The listing builds one solid part. Answer for the finished solid, in the listing's coordinates (mm). Face numbers are marked on the shaded views. A direction names the side the tool comes from. Give positions to 0.01 mm unless a question says otherwise; leave off trailing zeros. Write each loop counter-clockwise with the first axis right and the second up, starting at its lowest first coordinate (ties: lowest second). Pieces come first, ordered by that corner, then holes. Notation, with made-up numbers: M 83.25,31.5 L 105.25,31.5 A7 cw 105.25,38.5 Z; hole C 75,-27.5 d3. An arc over 180 degrees is marked long. Return JSON: item names as keys, results as strings.
from build123d import *

# Parameters (mm, degrees)
SKETCH1_W                                            = 59.1
SKETCH1_H                                            = 59.1
BOSS_EXTRUDE1_DEPTH                                  = 59.1
CUT_EXTRUDE1_START                                   = -2.25
SKETCH2_W                                            = 116.357411776
SKETCH2_H                                            = 94.431830133
CUT_EXTRUDE1_DEPTH                                   = 71.232302632
FILLET1_R                                            = 7.5
SHELL1_T                                             = -2.5
CUT_EXTRUDE7_DEPTH                                   = 35
BOSS_EXTRUDE2_START                                  = 3
SKETCH18_R                                           = 5
BOSS_EXTRUDE2_DEPTH                                  = 3
SKETCH17_R                                           = 1.5
CUT_EXTRUDE10_DEPTH                                  = 10
CUT_EXTRUDE11_REACH                                  = 90.65
CSK_SLOT_FOR_M2_COUNTERSUNK_FLAT_HEAD_SC_D           = 2.4
CSK_SLOT_FOR_M2_COUNTERSUNK_FLAT_HEAD_SC_CSINK_D     = 4.4
CSK_SLOT_FOR_M2_COUNTERSUNK_FLAT_HEAD_SC_CSINK_ANGLE = 90
CSK_SLOT_FOR_M2_COUNTERSUNK_FLAT_HEA_2_D             = 2.4
CSK_SLOT_FOR_M2_COUNTERSUNK_FLAT_HEA_2_CSINK_D       = 4.4
CSK_SLOT_FOR_M2_COUNTERSUNK_FLAT_HEA_2_CSINK_ANGLE   = 90
CSK_SLOT_FOR_M2_COUNTERSUNK_FLAT_HEA_3_D             = 2.4
CSK_SLOT_FOR_M2_COUNTERSUNK_FLAT_HEA_3_CSINK_D       = 4.4
CSK_SLOT_FOR_M2_COUNTERSUNK_FLAT_HEA_3_CSINK_ANGLE   = 90
BOSS_EXTRUDE3_DEPTH                                  = 35
SKETCH28_W                                           = 7.5
SKETCH28_H                                           = 5.1
CUT_EXTRUDE12_DEPTH                                  = 62.984090748
SKETCH29_W                                           = 27.5
SKETCH29_H                                           = 5
BOSS_EXTRUDE4_DEPTH                                  = 5


with BuildPart() as part:
    # Sketch1 → Boss-Extrude1 (new body)
    with BuildSketch(Plane.XY):
        Rectangle(SKETCH1_W, SKETCH1_H)
    extrude(amount=BOSS_EXTRUDE1_DEPTH)

    # Sketch2 → Cut-Extrude1 (cut, through all)
    with BuildSketch(Plane(origin=(-13.400446417, -13.400446417, 19.55), x_dir=(0.9659258262890684, -0.2588190451025203, 0), z_dir=(0, 0, 1)).offset(CUT_EXTRUDE1_START)):
        with Locations((15.241895832, 15.980077556)):
            Rectangle(SKETCH2_W, SKETCH2_H)
    extrude(amount=-CUT_EXTRUDE1_DEPTH, mode=Mode.SUBTRACT)

    # Fillet1
    fillet1_edges = [part.edges().sort_by_distance(p)[0] for p in [
        (29.55, 0, 59.1),
        (0, 29.55, 59.1),
        (-29.55, 0, 59.1),
        (0, -29.55, 59.1),
        (-29.55, 29.55, 38.2),
        (29.55, 29.55, 38.2),
        (29.55, -29.55, 38.2),
        (-29.55, -29.55, 38.2),
    ]]
    fillet(fillet1_edges, radius=FILLET1_R)

    # Shell1
    shell1_openings = [part.faces().sort_by_distance(p)[0] for p in [
        (0, 0, 17.3),
    ]]
    offset(amount=SHELL1_T, openings=shell1_openings, kind=Kind.INTERSECTION)

    # Sketch14 → Cut-Extrude7 (cut)
    with BuildSketch(Plane.XY.offset(59.1)):
        Polygon((-29.55, -8.7), (-27.05, -8.7), (-27.05, -7.5), (-24.55, -7.5), (-24.55, -12.5), (-27.05, -12.5), (-27.05, -11.3), (-29.55, -11.3), align=None)
        Polygon((-29.55, 11.3), (-29.55, 8.7), (-27.05, 8.7), (-27.05, 7.5), (-24.55, 7.5), (-24.55, 12.5), (-27.05, 12.5), (-27.05, 11.3), align=None)
    extrude(amount=-CUT_EXTRUDE7_DEPTH, mode=Mode.SUBTRACT)

    # Sketch18 → Boss-Extrude2 (add)
    with BuildSketch(Plane(origin=(0, -27.05, 0), x_dir=(1, 0, 0), z_dir=(0, 1, 0)).offset(BOSS_EXTRUDE2_START)):
        with Locations((-22.05, -51.6)):
            Circle(SKETCH18_R)
    extrude(amount=-BOSS_EXTRUDE2_DEPTH)

    # Sketch17 → Cut-Extrude10 (cut)
    with BuildSketch(Plane.XZ.offset(29.55)):
        with Locations(Location((-22.05, 51.6, 0), (0, 0, 90))):
            Circle(SKETCH17_R)
    extrude(amount=-CUT_EXTRUDE10_DEPTH, mode=Mode.SUBTRACT)

    # Sketch20 → Cut-Extrude11 (cut, up to next)
    with BuildSketch(Plane.XZ.offset(29.55), mode=Mode.PRIVATE) as cut_extrude11_sk1:
        with BuildLine():
            Line((-22.647878988, 52.975696447), (-23.072143057, 53.399960516))
            Line((-23.072143057, 53.399960516), (-23.849960516, 52.622143057))
            Line((-23.849960516, 52.622143057), (-23.425696447, 52.197878988))
            ThreePointArc((-23.425696447, 52.197878988), (-23.110660172, 52.660660172), (-22.647878988, 52.975696447))
        make_face()
    cut_extrude11_tool1 = extrude(cut_extrude11_sk1.sketch, amount=-CUT_EXTRUDE11_REACH, mode=Mode.PRIVATE) & part.part
    # Sketch20 → Cut-Extrude11 (cut, up to next)
    with BuildSketch(Plane.XZ.offset(29.55), mode=Mode.PRIVATE) as cut_extrude11_sk2:
        with BuildLine():
            Line((-21.027856943, 49.800039484), (-21.452121012, 50.224303553))
            ThreePointArc((-21.452121012, 50.224303553), (-20.989339828, 50.539339828), (-20.674303553, 51.002121012))
            Line((-20.674303553, 51.002121012), (-20.250039484, 50.577856943))
            Line((-20.250039484, 50.577856943), (-21.027856943, 49.800039484))
        make_face()
    cut_extrude11_tool2 = extrude(cut_extrude11_sk2.sketch, amount=-CUT_EXTRUDE11_REACH, mode=Mode.PRIVATE) & part.part
    add(cut_extrude11_tool1.solids().sort_by_distance((-23.27308, -29.55, 52.82308))[0], mode=Mode.SUBTRACT)
    add(cut_extrude11_tool2.solids().sort_by_distance((-20.82692, -29.55, 50.37692))[0], mode=Mode.SUBTRACT)

    # CSK SLOT for M2 Countersunk Flat Head Sc (through all)
    with Locations(Plane.ZX.offset(29.55)):
        with Locations((29.55, 0)):
            CounterSinkHole(CSK_SLOT_FOR_M2_COUNTERSUNK_FLAT_HEAD_SC_D / 2, CSK_SLOT_FOR_M2_COUNTERSUNK_FLAT_HEAD_SC_CSINK_D / 2, counter_sink_angle=CSK_SLOT_FOR_M2_COUNTERSUNK_FLAT_HEAD_SC_CSINK_ANGLE)

    # CSK SLOT for M2 Countersunk Flat Hea 2 (through all)
    with Locations(Plane.XY.offset(59.1)):
        with Locations((0, 0)):
            CounterSinkHole(CSK_SLOT_FOR_M2_COUNTERSUNK_FLAT_HEA_2_D / 2, CSK_SLOT_FOR_M2_COUNTERSUNK_FLAT_HEA_2_CSINK_D / 2, counter_sink_angle=CSK_SLOT_FOR_M2_COUNTERSUNK_FLAT_HEA_2_CSINK_ANGLE)

    # CSK SLOT for M2 Countersunk Flat Hea 3 (through all)
    with Locations(Plane(origin=(0, -29.55, 0), x_dir=(-1, 0, 0), z_dir=(0, -1, 0))):
        with Locations((0, -29.55)):
            CounterSinkHole(CSK_SLOT_FOR_M2_COUNTERSUNK_FLAT_HEA_3_D / 2, CSK_SLOT_FOR_M2_COUNTERSUNK_FLAT_HEA_3_CSINK_D / 2, counter_sink_angle=CSK_SLOT_FOR_M2_COUNTERSUNK_FLAT_HEA_3_CSINK_ANGLE)

    # Sketch27 → Boss-Extrude3 (add)
    with BuildSketch(Plane(origin=(-29.55, 29.55, 0), x_dir=(0, 0, -1), z_dir=(1, 0, 0))):
        Polygon((-18.3, -59.1), (-18.3, -61.7), (-17.05, -61.7), (-17.05, -64.2), (-22.05, -64.2), (-22.05, -61.7), (-20.8, -61.7), (-20.8, -59.1), align=None)
        Polygon((-38.3, -59.1), (-40.8, -59.1), (-40.8, -61.7), (-42.05, -61.7), (-42.05, -64.2), (-37.05, -64.2), (-37.05, -61.7), (-38.3, -61.7), align=None)
    extrude(amount=BOSS_EXTRUDE3_DEPTH)

    # Sketch28 → Cut-Extrude12 (cut, through all)
    with BuildSketch(Plane.XY.offset(59.1)):
        with Locations((-25.8, -32.1)):
            Rectangle(SKETCH28_W, SKETCH28_H)
    extrude(amount=-CUT_EXTRUDE12_DEPTH, mode=Mode.SUBTRACT)

    # Sketch29 → Boss-Extrude4 (add)
    with BuildSketch(Plane.XY.offset(59.1)):
        with Locations((8.3, -10)):
            Rectangle(SKETCH29_W, SKETCH29_H)
        with Locations((8.3, 10)):
            Rectangle(SKETCH29_W, SKETCH29_H)
    extrude(amount=BOSS_EXTRUDE4_DEPTH)


solid = part.part
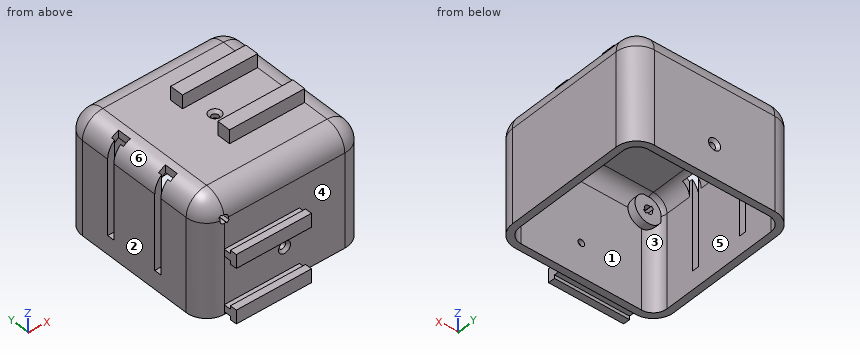
Item 1: Which of the six approach directions +Z, -Z, +X, -X, +Y, -Y give full straight-line access (tool end or side, diameter ignored) to the marked faces 1 and 2?
Geometry results:
{"face 1": "-Z", "face 2": "+Z, -Z, -X, +Y, -Y"}
Item 2: Given pin 1 Ø3 at (x, z) = (0, 29.55) entering from -Y; pin 2 Ø2 at (x, y) = (19.5, -26.5) entering from -Z; pin 3 Ø4 at (x, z) = (-4.5, 51) entering from -Y, each flat-ended and moving along its own axis, determine where each tip first touches the part or whether it passes through.
Geometry results:
{"pin 1": "stops at y = -28.85", "pin 2": "stops at z = 17.3", "pin 3": "stops at y = -29.55"}
Item 3: Determine the mould class of the marked faces 3, 4, 5 and 6 for opening direction X: +X half, -X half, draft (parallel to the pull), parting line (faces both ways), or undercut.
Geometry results:
{"face 3": "undercut", "face 4": "draft", "face 5": "undercut", "face 6": "-X half"}
Item 4: A cutting plane is placed at C-C, the plane x = -15.5. Write down the section's boundary in (y, z).
Geometry results:
{"outline": "M -34.65,17.05 L -32.15,17.05 L -32.15,18.3 L -29.55,18.3 L -29.55,17.3 L -27.05,17.3 L -27.05,51.6 A5 cw -22.05,56.6 L 22.05,56.6 A5 cw 27.05,51.6 L 27.05,17.3 L 29.55,17.3 L 29.55,51.6 A7.5 ccw 22.05,59.1 L -22.05,59.1 A7.5 ccw -29.55,51.6 L -29.55,40.8 L -32.15,40.8 L -32.15,42.05 L -34.65,42.05 L -34.65,37.05 L -32.15,37.05 L -32.15,38.3 L -29.55,38.3 L -29.55,20.8 L -32.15,20.8 L -32.15,22.05 L -34.65,22.05 Z"}
Item 5: A cutting plane is placed at A-A, the plane z = 44. Write down the section's boundary in (x, y), plus the area to 3 significant figures.
Geometry results:
{"outline": "M -29.55,-22.05 A7.5 ccw -22.05,-29.55 L 22.05,-29.55 A7.5 ccw 29.55,-22.05 L 29.55,22.05 A7.5 ccw 22.05,29.55 L -22.05,29.55 A7.5 ccw -29.55,22.05 L -29.55,11.3 L -27.05,11.3 L -27.05,22.05 A5 cw -22.05,27.05 L 22.05,27.05 A5 cw 27.05,22.05 L 27.05,-22.05 A5 cw 22.05,-27.05 L -22.05,-27.05 A5 cw -27.05,-22.05 L -27.05,-11.3 L -29.55,-11.3 Z; M -29.55,-8.7 L -27.05,-8.7 L -27.05,8.7 L -29.55,8.7 Z", "area": "526 mm2"}
Item 6: Find the intervals of material crossed by line 1 (Y direction, x = -21, z = 38); line 2 (X direction, y = 8, z = 38), in increasing order.
Geometry results:
{"line 1": "y = -34.65 to -32.15, -29.55 to -27.05, 27.05 to 29.55", "line 2": "x = -29.55 to -27.05, 27.05 to 29.55"}
Item 7: A cutting plane is placed at D-D, the plane x = 0. Count the separate pieces of the cut face and the enclosed holes in it, plus the area to 3 significant figures.
Geometry results:
{"separate pieces": "4", "enclosed holes": "0", "area": "398 mm2"}
Item 8: A cutting plane is placed at B-B, the plane y = -4. Write down the section's boundary in (x, z), plus the area to 3 significant figures.
Geometry results:
{"outline": "M -29.55,17.3 L -27.05,17.3 L -27.05,51.6 A5 cw -22.05,56.6 L 22.05,56.6 A5 cw 27.05,51.6 L 27.05,17.3 L 29.55,17.3 L 29.55,51.6 A7.5 ccw 22.05,59.1 L -22.05,59.1 A7.5 ccw -29.55,51.6 Z", "area": "331 mm2"}
